The listing builds one solid part. Answer for the finished solid, in the listing's coordinates (mm). Coordinates: 2 decimals unless noted, no trailing zeros. Write each loop counter-clockwise with the first axis right and the second up, starting at its lowest first coordinate (ties: lowest second). Pieces come first, ordered by that corner, then holes.
Autodesk Inventor part; units mm, degrees
ref_plane "YZ Plane" through (0, 0, 0) normal (1, 0, 0) x (0, 1, 0)
ref_plane "XZ Plane" through (0, 0, 0) normal (0, 1, 0) x (-1, 0, 0)
ref_plane "XY Plane" through (0, 0, 0) normal (0, 0, 1) x (1, 0, 0)
sketch "スケッチ1" plane through (0, 0, 0) normal (0, 0, 1) x (1, 0, 0)
  circle A0 centre (0, 0) radius 28.5
  line L0 (0, 0) -> (59.55, 0)
  line L1 (59.55, 0) -> (42.05, 0)
  line L2 (42.05, 0) -> (42.05, -70)
  line L3 (42.05, -70) -> (59.55, -70)
  line L4 (59.55, -70) -> (59.55, 0)
  line L5 (77.05, 0) -> (77.05, -70)
  line L6 (77.05, -70) -> (59.55, -70)
  line L7 (77.05, 0) -> (59.55, 0)
  line L8 (42.05, -70) -> (-17.7725, -22.2798)
  line L9 (77.05, -20) -> (42.05, -20)
  line L10 (77.05, -20) -> (16.5623, 23.1936)
  point P0 (42.05, 0)
  point P1 (28.5, 0)
  dimension "d0" = 57
  dimension "d1" = 59.55
  dimension "d2" = 17.5
  dimension "d3" = 70
  dimension "d31" = 50
extrude "押し出し1" add sketch "スケッチ1" along normal blind 2 contours A0 | L0 L2 L8 A0 | A0 L10 L0 | L0 L10 L4 L9 L2 | L2 L9 L4 L3 | L10 L9 L4 | L4 L9 L5 L6
sketch "スケッチ2" plane through (0, 0, 0) normal (0, 0, -1) x (-1, 0, 0)
  circle A0 centre (0, 0) radius 18.5
  dimension "d6" = 37
extrude "押し出し2" cut sketch "スケッチ2" against normal blind 2
sketch "スケッチ3" plane through (0, 0, 0) normal (0, 0, -1) x (-1, 0, 0)
  arc A0 (17.7725, -22.2798) -> (-16.5623, 23.1936) centre (0, 0) ccw
  circle A1 centre (0, 0) radius 25
  line L0 (0, 0) -> (0, 28.5)
  line L1 (0, 0) -> (12.5, 21.6506)
  point P0 (-19.257, 34.2013)
  point P1 (12.5, 21.6506)
  point P2 (-12.5, 21.6506)
  point P3 (-25, 0)
  point P4 (-12.5, -21.6506)
  point P5 (12.5, -21.6506)
  point P6 (25, 0)
  point P7 (-39.25, 0)
  dimension "d9" = 50
  dimension "d12" = 360
  dimension "d47" = 30
hole "穴1" at (-12.5, 21.6506, 0) at (12.5, 21.6506, 0) at (25, 0, 0) at (12.5, -21.6506, 0) at (-12.5, -21.6506, 0) at (-25, 0, 0) direction (0, 0, 1) diameter 3.2 end through all
sketch "スケッチ4" plane through (0, 0, 0) normal (0, 0, -1) x (-1, 0, 0)
  line L0 (-77.05, -70) -> (-77.05, -20)
  line L1 (17.7725, -22.2798) -> (-42.05, -70)
  line L2 (-42.05, -70) -> (-82.05, -70)
  line L3 (-77.05, -20) -> (-42.05, -20)
  line L4 (-42.05, -20) -> (-42.05, -70)
  line L5 (-42.05, -70) -> (-77.05, -70)
  line L6 (-77.05, -70) -> (-77.05, -20)
  line L7 (-59.55, -20) -> (-59.55, -70)
  point P0 (0, 0)
  point P1 (-59.55, -40)
  point P2 (-59.55, -60)
  dimension "d32" = 20
  dimension "d33" = 20
hole "穴2" at (59.55, -40, 0) at (59.55, -60, 0) direction (0, 0, 1) diameter 3.2 end through all
sketch "スケッチ5" plane through (0, 0, 0) normal (0, 0, -1) x (-1, 0, 0)
  arc A0 (17.7725, -22.2798) -> (-16.5623, 23.1936) centre (0, 0) ccw
  circle A1 centre (0, 0) radius 28.5
  line L0 (0, -28.5) -> (-42.05, -28.5)
  line L1 (17.7725, -22.2798) -> (-42.05, -70)
  line L2 (-42.05, -28.5) -> (-42.05, -70)
  point P0 (17.7725, -22.2798)
  point P1 (-2.7683, -39.25)
  point P2 (-16.5623, 23.1936)
  point P3 (17.7725, -22.2798)
  dimension "d35" = 57
extrude "押し出し3" cut sketch "スケッチ5" against normal blind 2 contours L1 L2 L0 A1
fillet "フィレット2" radius 20 1 edges at (42.05, -28.5, 1)
fillet "フィレット3" radius 5 3 edges at (42.05, -70, 1) (77.05, -70, 1) (77.05, -20, 1)
sketch "スケッチ6" plane through (0, 0, 0) normal (0, 0, -1) x (-1, 0, 0)
  circle A0 centre (12.5, 21.6506) radius 1.6
  circle A1 centre (12.5, 21.6506) radius 3
  circle A2 centre (-12.5, 21.6506) radius 3
  circle A3 centre (-25, 0) radius 3
  circle A4 centre (-12.5, -21.6506) radius 3
  circle A5 centre (12.5, -21.6506) radius 3
  circle A6 centre (25, 0) radius 3
  point P0 (0, 0)
  dimension "d40" = 6
  dimension "d43" = 360
extrude "押し出し4" [suppressed]
equation "\"d1\" = Sside"
equation "\"BendRadius\" = Thickness"
equation "\"BendReliefWidth\" = Thickness"
equation "\"BendReliefDepth\" = 0.5 * Thickness"
equation "\"CornerReliefSize\" = 4 * Thickness"
equation "\"MinimumRemnant\" = 2 * Thickness"
equation "\"TransitionRadius\" = BendRadius"
equation "\"JacobiRadiusSize\" = BendRadius"
equation "\"GapSize\" = Thickness"
properties part number "upperarm_fixplate1_forR0" material "アルミニウム 6061"
1. Section A-A on x = 12.5 is taken. Give the vertices of the cut face in (y, z).
Results found:
outline: (-28.5, 0) - (-23.25, 0) - (-23.25, 2) - (-28.5, 2) - close; (-20.05, 0) - (-13.64, 0) - (-13.64, 2) - (-20.05, 2) - close; (13.64, 0) - (20.05, 0) - (20.05, 2) - (13.64, 2) - close; (23.25, 0) - (25.61, 0) - (25.61, 2) - (23.25, 2) - close
2. A flat-ended cylindrical pin translates along its axis: P1, Ø5, axis at x = -12.5, y = -21.65, coming from the +Z side. Find the tip coordinate at first contact, or state that the pin passes through.
Results found:
P1: stops at z = 2
3. Section C-C on y = 0 is taken. Give the vertices of the cut face in (x, z), then the cut area to 3 significant figures.
Results found:
outline: (-28.5, 0) - (-26.6, 0) - (-26.6, 2) - (-28.5, 2) - close; (-23.4, 0) - (-18.5, 0) - (-18.5, 2) - (-23.4, 2) - close; (18.5, 0) - (23.4, 0) - (23.4, 2) - (18.5, 2) - close; (26.6, 0) - (49.04, 0) - (49.04, 2) - (26.6, 2) - close
area: 68.3 mm2
4. Section B-B on y = -60 is taken. Give the vertices of the cut face in (x, z), then the cut area to 3 significant figures.
Results found:
outline: (42.05, 0) - (57.95, 0) - (57.95, 2) - (42.05, 2) - close; (61.15, 0) - (77.05, 0) - (77.05, 2) - (61.15, 2) - close
area: 63.6 mm2
5. Section D-D on z = 1.25 is taken. State how many separate pieces and enclosed holes the cut face has, then the cut area to 3 significant figures.
Results found:
separate pieces: 1
enclosed holes: 9
area: 4,400 mm2
6. Find the intervals of material crossed by L1, parallel to Y at x = 59.55, z = 0.55; L2, parallel to X at y = -1, z = 1.9; L3, parallel to Y at x = 0, z = 1.1, in increasing order.
Results found:
L1: y = -70 to -61.6, -58.4 to -41.6, -38.4 to -7.5
L2: x = -28.48 to -26.25, -23.75 to -18.47, 18.47 to 23.75, 26.25 to 50.44
L3: y = -28.5 to -18.5, 18.5 to 28.5
7. For a pull along Y with two mould halves and no side action, classify faces 1 (the cylindrical face through (-24.03, -1.27, 1.01)), 2 (the flat face through (35, -20, 0)), 3 (the cylindrical face through (36.347, -34.514, 1.014)) as pulls with the +Y half, pulls with the -Y half, needs draft (parallel to the pull), parting line crosses it, or undercut.
Results found:
face 1: undercut
face 2: needs draft
face 3: pulls with the -Y half
